CAD build for the part. Positions are in the model's coordinates, mm. Give positions to 0.01 mm unless a question says otherwise; leave off trailing zeros. Order: outer loops, then holes, each group sorted by start corner. A loop starts at its lowest first (then second) coordinate and runs counter-clockwise, first axis right, second up.
```python
from build123d import *

# Parameters (mm, degrees)
SKETCH1_W            = 25
SKETCH1_H            = 25
SKETCH1_R            = 5
BOSS_EXTRUDE2_DEPTH  = 2
FILLET2_R            = 2
M3_CLEARANCE_HOLE1_D = 3.4


with BuildPart() as part:
    # Sketch1 → Boss-Extrude2 (new body)
    with BuildSketch(Plane.XY):
        Rectangle(SKETCH1_W, SKETCH1_H)
        Circle(SKETCH1_R, mode=Mode.SUBTRACT)
    extrude(amount=BOSS_EXTRUDE2_DEPTH)

    # Fillet2
    fillet2_edges = [part.edges().sort_by_distance(p)[0] for p in [
        (-12.5, 12.5, 1),
        (12.5, 12.5, 1),
        (12.5, -12.5, 1),
        (-12.5, -12.5, 1),
    ]]
    fillet(fillet2_edges, radius=FILLET2_R)

    # M3 Clearance Hole1 (through all)
    with Locations(Plane.XY.offset(2)):
        with Locations((-6.717514421, 6.717514421), (5.656854249, 5.656854249), (6.717514421, -6.717514421), (-5.656854249, -5.656854249)):
            Hole(M3_CLEARANCE_HOLE1_D / 2)


solid = part.part
```
Item 1: Slice it at A-A (x = 0). Give the cut face in (y, z).
Item 2: Drop a flat-ended pin along its axis: pin 1 Ø2 at (x, y) = (-6.72, 6.72) entering from -Z. Give the stop position or say it passes through.
Item 3: Slice it at C-C (x = -4.25). Give the cut face in (y, z).
Item 4: Wall check: L1, parallel to X at y = 5.75, z = 0.9; L2, parallel to Y at x = 4.5, z = 0.35; L3, parallel to X at y = -6.75, z = 0.4. Give the ranges that are in metal, low to high.
Item 5: Two-plate mould, pull along X, no slides. Class faces 1 (the face through (5.4, 0.2, 2)), 2 (the face through (12.5, 0, 1)), 3 (the face through (8.416, -6.643, 0.986)): released by +X, released by -X, zero draft, split by the parting line, or undercut.
Item 6: Slice it at D-D (z = 1.55). Give the cut face in (x, y).
A:
1. outline: (-12.5, 0) - (-5, 0) - (-5, 2) - (-12.5, 2) - close; (5, 0) - (12.5, 0) - (12.5, 2) - (5, 2) - close
2. pin 1: passes through
3. outline: (-12.5, 0) - (-6.61, 0) - (-6.61, 2) - (-12.5, 2) - close; (-4.7, 0) - (-2.63, 0) - (-2.63, 2) - (-4.7, 2) - close; (2.63, 0) - (12.5, 0) - (12.5, 2) - (2.63, 2) - close
4. L1: x = -12.5 to -8.12, -5.32 to 3.96, 7.35 to 12.5
4. L2: y = -12.5 to -2.18, 2.18 to 4.41, 6.9 to 12.5
4. L3: x = -12.5 to -6.96, -4.35 to 5.02, 8.42 to 12.5
5. face 1: zero draft
5. face 2: released by +X
5. face 3: undercut
6. outline: (-12.5, -10.5) arc R2 ccw to (-10.5, -12.5) - (10.5, -12.5) arc R2 ccw to (12.5, -10.5) - (12.5, 10.5) arc R2 ccw to (10.5, 12.5) - (-10.5, 12.5) arc R2 ccw to (-12.5, 10.5) - close; hole circle Ø3.4 at (-6.72, 6.72); hole circle Ø3.4 at (-5.66, -5.66); hole circle Ø10 at (0, 0); hole circle Ø3.4 at (5.66, 5.66); hole circle Ø3.4 at (6.72, -6.72)
